from build123d import *

# Parameters (mm, degrees)
SKETCH1_W           = 11.999999876
SKETCH1_H           = 11.999999876
BOSS_EXTRUDE1_DEPTH = 22.499999958
SKETCH2_R           = 5.499999922
BOSS_EXTRUDE2_DEPTH = 50.000000076
SKETCH3_W           = 11.999999876
SKETCH3_H           = 11.999999876
BOSS_EXTRUDE3_DEPTH = 11.999999876
SKETCH4_R           = 4.000000128
BOSS_EXTRUDE4_DEPTH = 8.000000002
CHAMFER1_SIZE       = 2.50000008
CHAMFER2_SIZE       = 2.50000008
SKETCH5_W           = 4.000000128
SKETCH5_H           = 12.999999908
CUT_EXTRUDE1_DEPTH  = 94.467908824
SKETCH6_R           = 2.049999964
CUT_EXTRUDE2_DEPTH  = 94.467908824
SKETCH7_R           = 2.250000072
CUT_EXTRUDE3_DEPTH  = 6.99999997
SKETCH8_R           = 2.250000072
CUT_EXTRUDE4_DEPTH  = 6.99999997


with BuildPart() as part:
    # Sketch1 → Boss-Extrude1 (new body)
    with BuildSketch(Plane(origin=(0, 0, 0), x_dir=(1, 0, 0), z_dir=(0, 1, 0))):
        Rectangle(SKETCH1_W, SKETCH1_H)
    extrude(amount=BOSS_EXTRUDE1_DEPTH)

    # Sketch2 → Boss-Extrude2 (add)
    with BuildSketch(Plane(origin=(0, 22.499999958, 0), x_dir=(1, 0, 0), z_dir=(0, 1, 0))):
        with Locations(Location((0, 0, 0), (0, 0, 270))):
            Circle(SKETCH2_R)
    extrude(amount=BOSS_EXTRUDE2_DEPTH)

    # Sketch3 → Boss-Extrude3 (add)
    with BuildSketch(Plane(origin=(0, 72.500000034, 0), x_dir=(1, 0, 0), z_dir=(0, 1, 0))):
        Rectangle(SKETCH3_W, SKETCH3_H)
    extrude(amount=BOSS_EXTRUDE3_DEPTH)

    # Sketch4 → Boss-Extrude4 (add)
    with BuildSketch(Plane(origin=(0, 84.49999991, 0), x_dir=(1, 0, 0), z_dir=(0, 1, 0))):
        with Locations(Location((0, 0, 0), (0, 0, 270))):
            Circle(SKETCH4_R)
    extrude(amount=BOSS_EXTRUDE4_DEPTH)

    # Chamfer1
    chamfer1_edges = [part.edges().sort_by_distance(p)[0] for p in [
        (5.999999938, 11.249999979, 5.999999938),
        (-5.999999938, 11.249999979, 5.999999938),
        (-5.999999938, 11.249999979, -5.999999938),
        (5.999999938, 11.249999979, -5.999999938),
    ]]
    chamfer(chamfer1_edges, length=CHAMFER1_SIZE)

    # Chamfer2
    chamfer2_edges = [part.edges().sort_by_distance(p)[0] for p in [
        (5.999999938, 78.499999972, 5.999999938),
        (5.999999938, 78.499999972, -5.999999938),
        (-5.999999938, 78.499999972, -5.999999938),
        (-5.999999938, 78.499999972, 5.999999938),
    ]]
    chamfer(chamfer2_edges, length=CHAMFER2_SIZE)

    # Sketch5 → Cut-Extrude1 (cut, through all)
    with BuildSketch(Plane.XY.offset(5.999999938)):
        with Locations((0, 6.499999954)):
            Rectangle(SKETCH5_W, SKETCH5_H)
    extrude(amount=-CUT_EXTRUDE1_DEPTH, mode=Mode.SUBTRACT)

    # Sketch6 → Cut-Extrude2 (cut, through all)
    with BuildSketch(Plane(origin=(5.999999938, 0, 0), x_dir=(0, 0, -1), z_dir=(1, 0, 0))):
        with Locations((0, 4.999999906)):
            Circle(SKETCH6_R)
    extrude(amount=-CUT_EXTRUDE2_DEPTH, mode=Mode.SUBTRACT)

    # Sketch7 → Cut-Extrude3 (cut)
    with BuildSketch(Plane.XY.offset(5.999999938)):
        with Locations((0, 17.749999806)):
            Circle(SKETCH7_R)
    extrude(amount=-CUT_EXTRUDE3_DEPTH, mode=Mode.SUBTRACT)

    # Sketch8 → Cut-Extrude4 (cut)
    with BuildSketch(Plane.XY.offset(5.999999938)):
        with Locations((0, 77.249999932)):
            Circle(SKETCH8_R)
    extrude(amount=-CUT_EXTRUDE4_DEPTH, mode=Mode.SUBTRACT)


solid = part.part
Design review of the part built by this model. Coordinates are the model's own, in mm. A direction names the side the tool comes from. Give positions to 0.01 mm unless a question says otherwise; leave off trailing zeros. Loops run counter-clockwise (first coordinate to the right, second up) from the corner with the lowest first, then second, coordinate; pieces in that order, holes last. Notation, with made-up numbers: (30, 60) - (50, 60) arc R37 cw to (50, 99) - close; hole circle Ø1 at (70, -4). An arc over 180 degrees is marked (long way). Use CSV: the item, a comma, the result in double quotes. Start each with the question number.
1. Wall thickness on L1, parallel to X at y = 77.25, z = 3.5; L2, parallel to Y at x = 2.9, z = 0; L3, parallel to Z at x = 3.2, y = 5: over which ranges is each line inside the solid? List them lowest first.
2. Draft analysis for pull direction Y (two halves, no side actions). For faces 6 (the flat face through (0, 13, 0)), 7 (the flat face through (3, 22.5, 5)), 8 (the flat face through (-6, 78, 0)), state which applies: released by +Y, released by -Y, zero draft, split by the parting line, or undercut.
3. Add section A-A (z = 0). Count the separate pieces of the cut face and the enclosed holes in it, plus the area to 3 significant figures.
4. Machinability: for faces 1 (the flat face through (0, 14, -6)), 2 (the flat face through (2, 8, 0)), 3 (the flat face through (-4.7, 78.4, 4.8)), 4 (the flat face through (0, 18, -1)), 5 (the flat face through (-1.42, 84.5, 3.92)), which of the approach directions +Z, -Z, +X, -X, +Y, -Y give a long, thin tool a straight path to every point of the face, cutting with its end or side? Answer none if there is none.
5. Add section C-C (x = 0). State the section outline as (y, z) points.
6. Add section D-D (y = 77.25). State the section outline as (x, z) points, plus the area to 4 significant figures.
7. Insertion check: P1, Ø4, axis at x = 0, y = 77.25, coming from the +Z side; P2, Ø1, axis at y = 28, z = 3.5, coming from the +X side; P3, Ø6, axis at y = 63.5, z = -2, coming from the +X side. Each pin has a flat end and moves straight along its axis. Give the tip position at first contact, or say it passes through.
8. Add section B-B (y = 5). State the section outline as (x, z) points, plus the area to 3 significant figures.
Results found:
1,L1,"x = -6 to -2.25, 2.25 to 6"
1,L2,"y = 0 to 2.95, 7.05 to 92.5"
1,L3,"z = -6 to -2.05, 2.05 to 6"
2,face 6,"released by -Y"
2,face 7,"undercut"
2,face 8,"zero draft"
3,separate pieces,"3"
3,enclosed holes,"2"
3,area,"911 mm²"
4,face 1,"-Z, +X, -X, +Y, -Y"
4,face 2,"+Z, -Z, -Y"
4,face 3,"+Z, -X, +Y, -Y"
4,face 4,"+Z"
4,face 5,"+Y"
5,outline,"(13, -6) - (22.5, -6) - (22.5, -5.5) - (72.5, -5.5) - (72.5, -6) - (84.5, -6) - (84.5, -4) - (92.5, -4) - (92.5, 4) - (84.5, 4) - (84.5, 6) - (79.5, 6) - (79.5, -1) - (75, -1) - (75, 6) - (72.5, 6) - (72.5, 5.5) - (22.5, 5.5) - (22.5, 6) - (20, 6) - (20, -1) - (15.5, -1) - (15.5, 6) - (13, 6) - close"
6,outline,"(-6, -3.5) - (-3.5, -6) - (3.5, -6) - (6, -3.5) - (6, 3.5) - (3.5, 6) - (2.25, 6) - (2.25, -1) - (-2.25, -1) - (-2.25, 6) - (-3.5, 6) - (-6, 3.5) - close"
6,area,"100.0 mm²"
7,P1,"stops at z = -1"
7,P2,"stops at x = 4.61"
7,P3,"stops at x = 5.5"
8,outline,"(-6, -3.5) - (-3.5, -6) - (-2, -6) - (-2, -2.05) - (-6, -2.05) - close; (-6, 2.05) - (-2, 2.05) - (-2, 6) - (-3.5, 6) - (-6, 3.5) - close; (2, -6) - (3.5, -6) - (6, -3.5) - (6, -2.05) - (2, -2.05) - close; (2, 2.05) - (6, 2.05) - (6, 3.5) - (3.5, 6) - (2, 6) - close"
8,area,"50.7 mm²"
